from build123d import *

# Parameters (mm, degrees)
SKETCH_W        = 89
SKETCH_H        = 56
SKETCH_W_2      = 76
SKETCH_H_2      = 42
PAD_DEPTH       = 1.5
SKETCH001_R     = 2.5
PAD001_DEPTH    = 3
SKETCH002_R     = 1.5
POCKET_DEPTH    = 4.501
FILLET_R        = 4
PAD002_DEPTH    = 1.5
SKETCH004_R     = 1.5
SKETCH004_R_2   = 1.15
POCKET001_DEPTH = 1.501
FILLET001_R     = 7


with BuildPart() as arduinosupport:
    # Sketch → Pad (new body)
    with BuildSketch(Plane.XY):
        with Locations((7.033953, -27.68594)):
            Rectangle(SKETCH_W, SKETCH_H)
        with Locations((7.033953, -27.68594)):
            Rectangle(SKETCH_W_2, SKETCH_H_2, mode=Mode.SUBTRACT)
    extrude(amount=PAD_DEPTH)

    # Sketch001 (on Face10 of Pad) → Pad001 (join)
    with BuildSketch(Plane.XY.offset(1.5)):
        with Locations((-33.016678, -3.147287)):
            Circle(SKETCH001_R)
        with Locations((-34.322529, -51.407287)):
            Circle(SKETCH001_R)
        with Locations((41.913322, -3.147287)):
            Circle(SKETCH001_R)
        with Locations((48.263322, -51.407287)):
            Circle(SKETCH001_R)
    extrude(amount=PAD001_DEPTH)

    # Sketch002 (on Face15 of Pad001) → Pocket (cut, through all)
    with BuildSketch(Plane.XY.offset(4.5)):
        with Locations((-33.016678, -3.147287)):
            Circle(SKETCH002_R)
        with Locations((-34.322529, -51.407287)):
            Circle(SKETCH002_R)
        with Locations((48.263322, -51.407287)):
            Circle(SKETCH002_R)
        with Locations((41.913322, -3.147287)):
            Circle(SKETCH002_R)
    extrude(amount=-POCKET_DEPTH, mode=Mode.SUBTRACT)

    # Fillet
    fillet_edges = [arduinosupport.edges().sort_by_distance(p)[0] for p in [
        (51.533953, 0.31406, 0.75),
        (51.533953, -55.68594, 0.75),
        (-37.466047, -55.68594, 0.75),
        (-37.466047, 0.31406, 0.75),
    ]]
    fillet(fillet_edges, radius=FILLET_R)


with BuildPart() as obj1:
    # Sketch003 → Pad002 (new body)
    with BuildSketch(Plane.XY):
        Polygon((12.977516, -66.941809), (-11.737781, -66.941809), (-21.072386, -57.607204), (-21.072386, 21.723586), (-11.737781, 31.058191), (12.977516, 31.058191), (22.312121, 21.723586), (22.312121, -57.607204), align=None)
        with BuildLine():
            Line((17.312121, 20.201021), (17.312121, 13.932858))
            Line((17.312121, 13.932858), (13.312121, 13.932858))
            ThreePointArc((13.312121, 13.932858), (11.272121, 11.892858), (13.312121, 9.852858))
            Line((17.312121, 9.852858), (13.312121, 9.852858))
            Line((17.312121, 9.852858), (17.312121, -56.084639))
            Line((17.312121, -56.084639), (12.454951, -60.941809))
            Line((12.454951, -60.941809), (-11.215216, -60.941809))
            Line((-11.215216, -60.941809), (-16.072386, -56.084639))
            Line((-16.072386, -56.084639), (-16.072386, 9.852858))
            Line((-12.072386, 9.852858), (-16.072386, 9.852858))
            ThreePointArc((-12.072386, 9.852858), (-10.032386, 11.892858), (-12.072386, 13.932858))
            Line((-16.072386, 13.932858), (-12.072386, 13.932858))
            Line((-16.072386, 20.201021), (-16.072386, 13.932858))
            Line((-11.215216, 25.058191), (-16.072386, 20.201021))
            Line((-11.215216, 25.058191), (12.454951, 25.058191))
            Line((12.454951, 25.058191), (17.312121, 20.201021))
        make_face(mode=Mode.SUBTRACT)
    extrude(amount=PAD002_DEPTH)

    # Sketch004 (on Face26 of Pad002) → Pocket001 (cut, through all)
    with BuildSketch(Plane.XY.offset(1.5)):
        with Locations((-7.589837, 27.917404)):
            Circle(SKETCH004_R)
        with Locations((7.410163, 27.917404)):
            Circle(SKETCH004_R)
        with Locations((-7.589837, -64.082596)):
            Circle(SKETCH004_R)
        with Locations((7.410163, -64.082596)):
            Circle(SKETCH004_R)
        with Locations((13.312121, 11.892858)):
            Circle(SKETCH004_R_2)
        with Locations((-12.072386, 11.892858)):
            Circle(SKETCH004_R_2)
    extrude(amount=-POCKET001_DEPTH, mode=Mode.SUBTRACT)

    # Fillet001
    fillet001_edges = [obj1.edges().sort_by_distance(p)[0] for p in [
        (12.977516, -66.941809, 0.75),
        (22.312121, -57.607204, 0.75),
        (-11.737781, -66.941809, 0.75),
        (-21.072386, -57.607204, 0.75),
        (-16.072386, -56.084639, 0.75),
        (17.312121, -56.084639, 0.75),
        (12.454951, -60.941809, 0.75),
        (-11.215216, -60.941809, 0.75),
        (-21.072386, 21.723586, 0.75),
        (-11.737781, 31.058191, 0.75),
        (22.312121, 21.723586, 0.75),
        (12.977516, 31.058191, 0.75),
        (-16.072386, 20.201021, 0.75),
        (-11.215216, 25.058191, 0.75),
        (12.454951, 25.058191, 0.75),
        (17.312121, 20.201021, 0.75),
    ]]
    fillet(fillet001_edges, radius=FILLET001_R)

    # Boolean: union ArduinoSupport
    add(arduinosupport.part)


solid = obj1.part
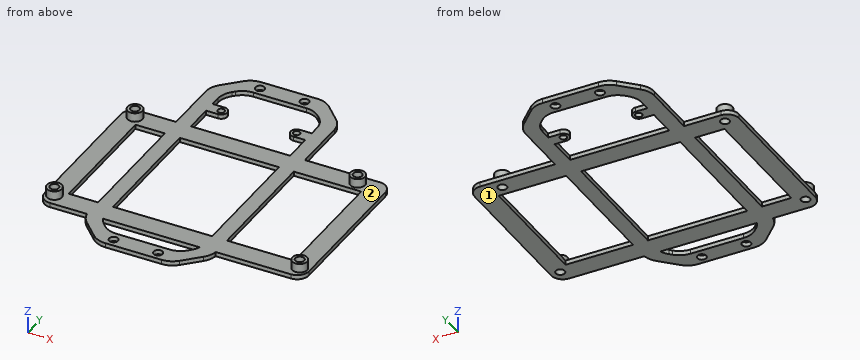
Read the model definition and answer for the solid it produces. Units are mm, in the model's axes. Face numbers are marked on the shaded views. Give positions to 0.01 mm unless a question says otherwise; leave off trailing zeros. Write each loop counter-clockwise with the first axis right and the second up, starting at its lowest first coordinate (ties: lowest second). Pieces come first, ordered by that corner, then holes. Notation, with made-up numbers: (-22.75, -1) -> (35.25, -1) arc R23 ccw to (35.25, 23) -> close; hole circle Ø1 at (66, -16.5). An arc over 180 degrees is marked (long way). Answer as a JSON object with one key per item and string values. Group by question number.
1) Each of these flat-tipped pins is pushed along its axis until it touches: P1, Ø1.6, axis at x = -28, z = 0.5, coming from the -Y side; P2, Ø1.6, axis at x = 14.5, z = 1, coming from the -Y side; P3, Ø0.8, axis at x = 36, z = 0.5, coming from the +Y side; P4, Ø8, axis at x = 40.5, y = -34.5, coming from the -Z side. Where does it stop, or does it pass through?
2) Find section D-D (x = 2). Write down the section's boundary in (y, z), and give its area (3 significant figures).
3) The mould has two halves that part along X. Classify the marked faces 1 and 2: +X half, -X half, draft (parallel to the pull), parting line (faces both ways), or undercut.
4) Find section C-C (z = 3.7). Write down the section's boundary in (x, y).
5) Consider L1, parallel to X at y = -41, z = 0.8; L2, parallel to X at y = -50.5, z = 3; L3, parallel to Y at x = 42.5, z = 1.15. Determine where each line is inside the solid, lowest interval first. Write a range as from..to.
6) Find section A-A (y = -46). Write down the section's boundary in (x, z).
7) Find section B-B (x = -25). Write down the section's boundary in (y, z), and give its area (3 significant figures).
Values follow:
{
 "1": {"P1": "stops at y = -55.69", "P2": "stops at y = -65.93", "P3": "stops at y = 0.31", "P4": "passes through"},
 "2": {"outline": "(-66.94, 0) -> (-60.94, 0) -> (-60.94, 1.5) -> (-66.94, 1.5) -> close; (-55.69, 0) -> (-48.69, 0) -> (-48.69, 1.5) -> (-55.69, 1.5) -> close; (-6.69, 0) -> (0.31, 0) -> (0.31, 1.5) -> (-6.69, 1.5) -> close; (25.06, 0) -> (31.06, 0) -> (31.06, 1.5) -> (25.06, 1.5) -> close", "area": "39.0 mm2"},
 "3": {"face 1": "draft", "face 2": "undercut"},
 "4": {"outline": "circle Ø5 at (-34.32, -51.41); circle Ø5 at (-33.02, -3.15); circle Ø5 at (41.91, -3.15); circle Ø5 at (48.26, -51.41); hole circle Ø3 at (-34.32, -51.41); hole circle Ø3 at (-33.02, -3.15); hole circle Ø3 at (41.91, -3.15); hole circle Ø3 at (48.26, -51.41)"},
 "5": {"L1": "x = -37.47..-30.97, -21.07..-16.07, 17.31..22.31, 45.03..51.53", "L2": "x = -36.65..-35.52, -33.13..-31.99, 45.93..47.07, 49.46..50.59", "L3": "y = -55.69..-48.69, -6.69..-4.53, -1.77..0.31"},
 "6": {"outline": "(-37.47, 0) -> (-30.97, 0) -> (-30.97, 1.5) -> (-37.47, 1.5) -> close; (-21.07, 0) -> (-16.07, 0) -> (-16.07, 1.5) -> (-21.07, 1.5) -> close; (17.31, 0) -> (22.31, 0) -> (22.31, 1.5) -> (17.31, 1.5) -> close; (45.03, 0) -> (51.53, 0) -> (51.53, 1.5) -> (45.03, 1.5) -> close"},
 "7": {"outline": "(-55.69, 0) -> (-48.69, 0) -> (-48.69, 1.5) -> (-55.69, 1.5) -> close; (-6.69, 0) -> (0.31, 0) -> (0.31, 1.5) -> (-6.69, 1.5) -> close", "area": "21.0 mm2"}
}
